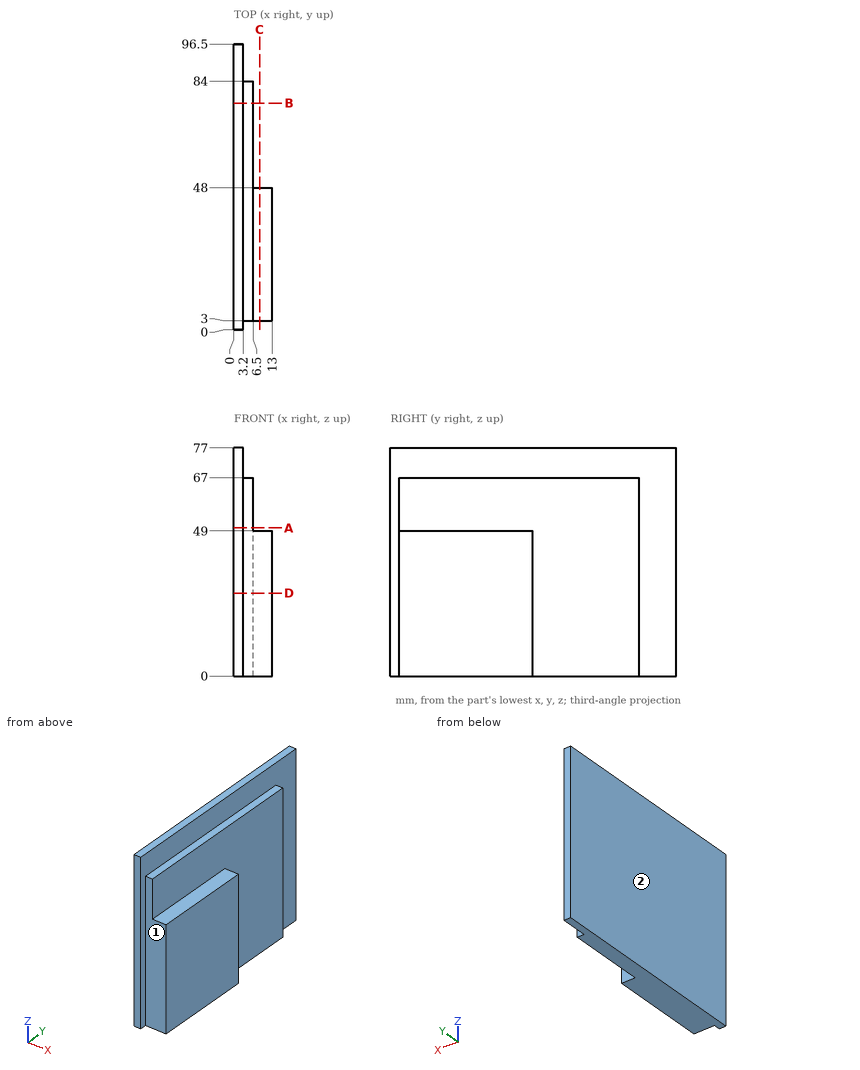
The figure shows three views and two pictorial views of one solid part (mm, origin at its lowest corner). Answer the questions. A direction names the side the tool comes from. Coordinates: 2 decimals unless noted, no trailing zeros. Loops run counter-clockwise (first coordinate to the right, second up) from the corner with the lowest first, then second, coordinate; pieces in that order, holes last. Notation, with made-up numbers: M 33.5,-25 L 44.5,-25 A21 ccw 44.5,13 Z; hole C 57,-21.75 d10. An arc over 180 degrees is marked long. Use CSV: the item, a comma, the result in double quotes. Start each with the question number.
(1) Find section C-C, the plane x = 8.75. Give the vertices of the cut face in (y, z).
(2) Find section D-D, the plane z = 28. Give the vertices of the cut face in (x, y), then the cut area to 3 significant figures.
(3) Find section B-B, the plane y = 76.5. Give the vertices of the cut face in (x, z), then the cut area to 4 significant figures.
(4) Given pin 1 Ø3 at (x, z) = (9, 19.5) entering from +Y; pin 2 Ø5 at (x, z) = (7, 39) entering from -Y; pin 3 Ø1.6 at (x, y) = (5, 36.5) entering from +Z, each flat-ended and moving along its own axis, determine where each tip first touches the part or whether it passes through.
(5) Consider line 1 (Y direction, x = 4.25, z = 37); line 2 (X direction, y = 13.5, z = 65.5); line 3 (Z direction, x = 11, y = 9). Determine where each line is inside the solid, lowest interval first.
(6) For the marked faces 1 and 2, determine the directions among +Z, -Z, +X, -X, +Y, -Y from which every point of the face is accessible in a straight line to the end or side of a thin tool.
(7) Find section A-A, the plane z = 50. Give the vertices of the cut face in (x, y), then the cut area to 3 significant figures.
Recorded:
1,outline,"M 3,0 L 48,0 L 48,49 L 3,49 Z"
2,outline,"M 0,0 L 3.2,0 L 3.2,3 L 13,3 L 13,48 L 6.5,48 L 6.5,84 L 3.2,84 L 3.2,96.5 L 0,96.5 Z"
2,area,"869 mm^2"
3,outline,"M 0,0 L 6.5,0 L 6.5,67 L 3.2,67 L 3.2,77 L 0,77 Z"
3,area,"467.5 mm^2"
4,pin 1,"stops at y = 48"
4,pin 2,"stops at y = 3"
4,pin 3,"stops at z = 67"
5,line 1,"y = 3 to 84"
5,line 2,"x = 0 to 6.5"
5,line 3,"z = 0 to 49"
6,face 1,"+Z, -Z, +X, -Y"
6,face 2,"+Z, -Z, -X, +Y, -Y"
7,outline,"M 0,0 L 3.2,0 L 3.2,3 L 6.5,3 L 6.5,84 L 3.2,84 L 3.2,96.5 L 0,96.5 Z"
7,area,"576 mm^2"
